Input: part model. Units: mm. Frame: model coordinates. Round coordinates to 2 decimals unless told otherwise and drop trailing zeros. Loops run counter-clockwise (first coordinate to the right, second up) from the corner with the lowest first, then second, coordinate; pieces in that order, holes last. Notation, with made-up numbers: M 46,-25 L 76,-25 A8 ccw 76,-15 Z; hole C 16,24.25 d5. An arc over 180 degrees is marked long. Put each result on its own line as item: value. Start each with the question number.
1) Line query: probe 1 along Z at (x, y) = (-24.5, 0.7); probe 2 along X at (y, z) = (1.4, 50.8); probe 3 along Z at (x, y) = (1.5, 2.1). Output: solid intervals per line, ascending.
2) Section C-C on y = 1.9. State how many separate pieces and enclosed holes the cut face has, plus the area to 3 significant figures.
3) Pin query (flat end, axial travel): pin 1 (1.5 mm diameter, centred on y = 2, z = 54, fed in from -X); pin 2 (1.5 mm diameter, centred on y = 1, z = -53.5, fed in from -X). Return the tip coordinate at first contact, or that it passes through.
4) Section A-A on z = 50.8. Output: boundary loops of the cut face in (x, y).
5) Section B-B on x = -2.5. Output: boundary loops of the cut face in (y, z).
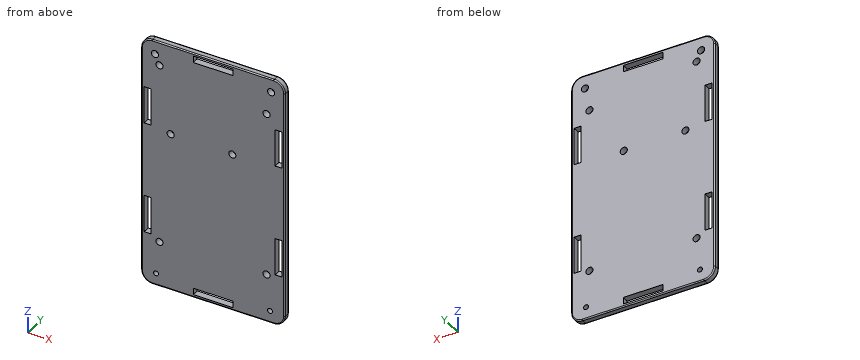
from build123d import *

# Parameters (mm, degrees)
BOSS_EXTRUDE3_DEPTH       = 3
SKETCH2_R                 = 1.608
CUT_EXTRUDE3_DEPTH        = 3
SKETCH7_R                 = 1.608
CUT_EXTRUDE8_DEPTH        = 3
SKETCH8_R                 = 1.608
CUT_EXTRUDE9_DEPTH        = 3
SKETCH9_R                 = 1.608
CUT_EXTRUDE11_DEPTH       = 3
SKETCH10_W                = 17.87
SKETCH10_H                = 3
SKETCH10_W_2              = 3
SKETCH10_H_2              = 16.933
CUT_EXTRUDE14_DEPTH       = 3
MIRROR4_COPY_1_SKETCH_W   = 17.87
MIRROR4_COPY_1_SKETCH_H   = 3
MIRROR4_COPY_1_SKETCH_W_2 = 3
MIRROR4_COPY_1_SKETCH_H_2 = 16.933
MIRROR4_COPY_1_DEPTH      = 3
SKETCH11_R                = 1.608
CUT_EXTRUDE15_DEPTH       = 3
FILLET1_R                 = 0.5
FILLET2_R                 = 0.5
SKETCH12_R                = 1.108
CUT_EXTRUDE16_DEPTH       = 3


with BuildPart() as part:
    # Sketch1 → Boss-Extrude3 (new body)
    with BuildSketch(Plane(origin=(0, 0, 0), x_dir=(1, 0, 0), z_dir=(0, 1, 0))):
        with BuildLine():
            Line((-32.5, -47), (-32.5, -52))
            ThreePointArc((-32.5, -52), (-31.035533906, -55.535533906), (-27.5, -57))
            Line((-27.5, -57), (-22.5, -57))
            Line((-22.5, -57), (22.5, -57))
            Line((22.5, -57), (27.5, -57))
            ThreePointArc((27.5, -57), (31.035533906, -55.535533906), (32.5, -52))
            Line((32.5, -52), (32.5, -47))
            Line((32.5, -47), (32.5, 47))
            Line((32.5, 47), (32.5, 52))
            ThreePointArc((32.5, 52), (31.035533906, 55.535533906), (27.5, 57))
            Line((27.5, 57), (22.5, 57))
            Line((22.5, 57), (-22.5, 57))
            Line((-22.5, 57), (-27.5, 57))
            ThreePointArc((-27.5, 57), (-31.035533906, 55.535533906), (-32.5, 52))
            Line((-32.5, 52), (-32.5, 47))
            Line((-32.5, 47), (-32.5, -47))
        make_face()
    extrude(amount=BOSS_EXTRUDE3_DEPTH)

    # Sketch2 → Cut-Extrude3 (cut)
    with BuildSketch(Plane(origin=(0, 3, 0), x_dir=(1, 0, 0), z_dir=(0, 1, 0))):
        with Locations(Location((24.261, 35.015, 0), (0, 0, 270))):
            Circle(SKETCH2_R)
    extrude(amount=-CUT_EXTRUDE3_DEPTH, mode=Mode.SUBTRACT)

    # Sketch7 → Cut-Extrude8 (cut)
    with BuildSketch(Plane.XZ):
        with Locations(Location((24.261, 39.945, 0), (0, 0, 270))):
            Circle(SKETCH7_R)
    extrude(amount=-CUT_EXTRUDE8_DEPTH, mode=Mode.SUBTRACT)

    # Sketch8 → Cut-Extrude9 (cut)
    with BuildSketch(Plane.XZ):
        with Locations(Location((-24.261, -36.285, 0), (0, 0, 270))):
            Circle(SKETCH8_R)
    extrude(amount=-CUT_EXTRUDE9_DEPTH, mode=Mode.SUBTRACT)

    # Sketch9 → Cut-Extrude11 (cut)
    with BuildSketch(Plane.XZ):
        with Locations(Location((-19.183, 15.745, 0), (0, 0, 270))):
            Circle(SKETCH9_R)
        with Locations(Location((8.725999982, 15.746, 0), (0, 0, 270))):
            Circle(SKETCH9_R)
        with Locations(Location((-24.261, 46.193, 0), (0, 0, 270))):
            Circle(SKETCH9_R)
    extrude(amount=-CUT_EXTRUDE11_DEPTH, mode=Mode.SUBTRACT)

    # Sketch10 → Cut-Extrude14 (cut)
    with BuildSketch(Plane(origin=(0, 3, 0), x_dir=(1, 0, 0), z_dir=(0, 1, 0))):
        with Locations((-0.005, -54.2)):
            Rectangle(SKETCH10_W, SKETCH10_H)
        with Locations((29.65, -25.3995)):
            Rectangle(SKETCH10_W_2, SKETCH10_H_2)
    cut_extrude14 = extrude(amount=-CUT_EXTRUDE14_DEPTH, mode=Mode.SUBTRACT)

    # Mirror3: Cut-Extrude14 across plane
    add(cut_extrude14.mirror(Plane.XY), mode=Mode.SUBTRACT)

    # Mirror4: Cut-Extrude14 across plane
    add(cut_extrude14.mirror(Plane(origin=(0, 0, 0), x_dir=(0, 0, 1), z_dir=(1, 0, 0))), mode=Mode.SUBTRACT)

    # Mirror4 copy 1 sketch → Mirror4 copy 1 (cut)
    with BuildSketch(Plane(origin=(0, 3, 0), x_dir=(-1, 0, 0), z_dir=(0, 1, 0))):
        with Locations((-0.005, -54.2)):
            Rectangle(MIRROR4_COPY_1_SKETCH_W, MIRROR4_COPY_1_SKETCH_H)
        with Locations((29.65, -25.3995)):
            Rectangle(MIRROR4_COPY_1_SKETCH_W_2, MIRROR4_COPY_1_SKETCH_H_2)
    extrude(amount=-MIRROR4_COPY_1_DEPTH, mode=Mode.SUBTRACT)

    # Sketch11 → Cut-Extrude15 (cut)
    with BuildSketch(Plane(origin=(0, 3, 0), x_dir=(1, 0, 0), z_dir=(0, 1, 0))):
        with Locations(Location((-26.3, -50.8, 0), (0, 0, 270))):
            Circle(SKETCH11_R)
    cut_extrude15 = extrude(amount=-CUT_EXTRUDE15_DEPTH, mode=Mode.SUBTRACT)

    # Mirror5: Cut-Extrude15 across plane
    add(cut_extrude15.mirror(Plane(origin=(0, 0, 0), x_dir=(0, 0, 1), z_dir=(1, 0, 0))), mode=Mode.SUBTRACT)

    # Fillet1
    fillet1_edges = [part.edges().sort_by_distance(p)[0] for p in [
        (0, 0, -57),
        (31.035533906, 0, -55.535533906),
        (32.5, 0, 0),
        (31.035533906, 0, 55.535533906),
        (0, 0, 57),
        (-31.035533906, 0, 55.535533906),
        (-32.5, 0, 0),
        (-31.035533906, 0, -55.535533906),
    ]]
    fillet(fillet1_edges, radius=FILLET1_R)

    # Fillet2
    fillet2_edges = [part.edges().sort_by_distance(p)[0] for p in [
        (-32.5, 3, 0),
        (-31.035533906, 3, 55.535533906),
        (0, 3, 57),
        (31.035533906, 3, 55.535533906),
        (32.5, 3, 0),
        (0, 3, -57),
        (31.035533906, 3, -55.535533906),
        (-31.035533906, 3, -55.535533906),
    ]]
    fillet(fillet2_edges, radius=FILLET2_R)

    # Sketch12 → Cut-Extrude16 (cut)
    with BuildSketch(Plane(origin=(0, 3, 0), x_dir=(1, 0, 0), z_dir=(0, 1, 0))):
        with Locations(Location((25.8, 51.5, 0), (0, 0, 270))):
            Circle(SKETCH12_R)
    cut_extrude16 = extrude(amount=-CUT_EXTRUDE16_DEPTH, mode=Mode.SUBTRACT)

    # Mirror8: Cut-Extrude16 across plane
    add(cut_extrude16.mirror(Plane(origin=(0, 0, 0), x_dir=(0, 0, 1), z_dir=(1, 0, 0))), mode=Mode.SUBTRACT)


solid = part.part
Geometry results:
1. probe 1: z = -57 to -37.88, -34.69 to 44.6, 47.78 to 57
1. probe 2: x = -32.5 to -27.91, -24.69 to 24.69, 27.91 to 32.5
1. probe 3: z = -57 to -55.7, -52.7 to 52.7, 55.7 to 57
2. separate pieces: 1
2. enclosed holes: 16
2. area: 7,010 mm²
3. pin 1: stops at x = -32.34
3. pin 2: stops at x = -32.44
4. outline: M -32.5,0.5 A0.5 ccw -32,0 L -27.91,0 L -27.91,3 L -32,3 A0.5 ccw -32.5,2.5 Z; M -24.69,0 L 24.69,0 L 24.69,3 L -24.69,3 Z; M 27.91,0 L 32,0 A0.5 ccw 32.5,0.5 L 32.5,2.5 A0.5 ccw 32,3 L 27.91,3 Z
5. outline: M 0,-56.5 A0.5 ccw 0.5,-57 L 2.5,-57 A0.5 ccw 3,-56.5 L 3,-55.7 L 0,-55.7 Z; M 0,-52.7 L 3,-52.7 L 3,52.7 L 0,52.7 Z; M 0,55.7 L 3,55.7 L 3,56.5 A0.5 ccw 2.5,57 L 0.5,57 A0.5 ccw 0,56.5 Z
